```python
from build123d import *

# Parameters (mm, degrees)
SKETCH1_R                                         = 57.5
BOSS_EXTRUDE1_DEPTH                               = 6.4
SKETCH2_W                                         = 25.525
SKETCH2_H                                         = 20.295
CUT_EXTRUDE1_DEPTH                                = 7.4
SKETCH3_W                                         = 4
SKETCH3_H                                         = 20.295
CUT_EXTRUDE2_DEPTH                                = 3
CUT_EXTRUDE3_DEPTH                                = 3
SKETCH5_R                                         = 1
CUT_EXTRUDE4_DEPTH                                = 7.4
CSK_FOR_8_FLAT_HEAD_SOCKET_CAP_SCREW1_D           = 4.9149
CSK_FOR_8_FLAT_HEAD_SOCKET_CAP_SCREW1_CSINK_D     = 9.1186
CSK_FOR_8_FLAT_HEAD_SOCKET_CAP_SCREW1_CSINK_ANGLE = 82
BOSS_EXTRUDE2_DEPTH                               = 6.4
FILLET1_R                                         = 2
SKETCH10_R                                        = 57.5
SKETCH10_R_2                                      = 54.5
BOSS_EXTRUDE3_DEPTH                               = 6.375
FILLET2_R                                         = 1


with BuildPart() as part:
    # Sketch1 → Boss-Extrude1 (new body)
    with BuildSketch(Plane(origin=(0, 0, 0), x_dir=(1, 0, 0), z_dir=(0, 1, 0))):
        Circle(SKETCH1_R)
        with BuildLine():
            Line((-17.49944642, 27), (17.49944642, 27))
            ThreePointArc((17.49944642, 27), (32.175, 0), (17.49944642, -27))
            Line((17.49944642, -27), (-17.49944642, -27))
            ThreePointArc((-17.49944642, -27), (-32.175, 0), (-17.49944642, 27))
        make_face(mode=Mode.SUBTRACT)
    extrude(amount=BOSS_EXTRUDE1_DEPTH)

    # Sketch2 → Cut-Extrude1 (cut, through all)
    with BuildSketch(Plane(origin=(0, 6.4, 0), x_dir=(1, 0, 0), z_dir=(0, 1, 0))):
        with Locations((0, 40.1475)):
            Rectangle(SKETCH2_W, SKETCH2_H)
        with Locations((0, -40.1475)):
            Rectangle(SKETCH2_W, SKETCH2_H)
    extrude(amount=-CUT_EXTRUDE1_DEPTH, mode=Mode.SUBTRACT)

    # Sketch3 → Cut-Extrude2 (cut)
    with BuildSketch(Plane.XZ):
        with Locations((14.7625, 40.1475)):
            Rectangle(SKETCH3_W, SKETCH3_H)
        with Locations((-14.7625, 40.1475)):
            Rectangle(SKETCH3_W, SKETCH3_H)
        with Locations((14.7625, -40.1475)):
            Rectangle(SKETCH3_W, SKETCH3_H)
        with Locations((-14.7625, -40.1475)):
            Rectangle(SKETCH3_W, SKETCH3_H)
    extrude(amount=-CUT_EXTRUDE2_DEPTH, mode=Mode.SUBTRACT)

    # Sketch4 → Cut-Extrude3 (cut)
    with BuildSketch(Plane.XZ):
        with BuildLine():
            Line((-19.770159359, 30.503496503), (-17.49944642, 27))
            ThreePointArc((-17.49944642, 27), (-32.175, 0), (-17.49944642, -27))
            Line((-17.49944642, -27), (-19.770159359, -30.503496503))
            ThreePointArc((-19.770159359, -30.503496503), (-36.35, 0), (-19.770159359, 30.503496503))
        make_face()
        with BuildLine():
            ThreePointArc((19.770159359, 30.503496503), (36.35, 0), (19.770159359, -30.503496503))
            Line((19.770159359, -30.503496503), (17.49944642, -27))
            ThreePointArc((17.49944642, -27), (32.175, 0), (17.49944642, 27))
            Line((17.49944642, 27), (19.770159359, 30.503496503))
        make_face()
    extrude(amount=-CUT_EXTRUDE3_DEPTH, mode=Mode.SUBTRACT)

    # Sketch5 → Cut-Extrude4 (cut, through all)
    with BuildSketch(Plane.XZ):
        with Locations((-33.941125497, 33.941125497)):
            Circle(SKETCH5_R)
        with Locations((33.941125497, 33.941125497)):
            Circle(SKETCH5_R)
        with Locations((33.941125497, -33.941125497)):
            Circle(SKETCH5_R)
        with Locations((-33.941125497, -33.941125497)):
            Circle(SKETCH5_R)
    extrude(amount=-CUT_EXTRUDE4_DEPTH, mode=Mode.SUBTRACT)

    # CSK for #8 Flat Head Socket Cap Screw1 (through all)
    with Locations(Plane(origin=(0, 6.4, 0), x_dir=(1, 0, 0), z_dir=(0, 1, 0))):
        with Locations((-33.941125497, 33.941125497), (33.941125497, 33.941125497), (33.941125497, -33.941125497), (-33.941125497, -33.941125497)):
            CounterSinkHole(CSK_FOR_8_FLAT_HEAD_SOCKET_CAP_SCREW1_D / 2, CSK_FOR_8_FLAT_HEAD_SOCKET_CAP_SCREW1_CSINK_D / 2, counter_sink_angle=CSK_FOR_8_FLAT_HEAD_SOCKET_CAP_SCREW1_CSINK_ANGLE)

    # Sketch9 → Boss-Extrude2 (add)
    with BuildSketch(Plane(origin=(0, 6.4, 0), x_dir=(1, 0, 0), z_dir=(0, 1, 0))):
        with BuildLine():
            Line((-17.49944642, 27), (17.49944642, 27))
            Line((17.49944642, 27), (9.178880504, 22.337651011))
            ThreePointArc((9.178880504, 22.337651011), (0, 24.15), (-9.178880504, 22.337651011))
            Line((-9.178880504, 22.337651011), (-17.49944642, 27))
        make_face()
        with BuildLine():
            Line((17.49944642, -27), (9.178880504, -22.337651011))
            ThreePointArc((9.178880504, -22.337651011), (0, -24.15), (-9.178880504, -22.337651011))
            Line((-9.178880504, -22.337651011), (-17.49944642, -27))
            Line((-17.49944642, -27), (17.49944642, -27))
        make_face()
    extrude(amount=-BOSS_EXTRUDE2_DEPTH)

    # Fillet1
    fillet1_edges = [part.edges().sort_by_distance(p)[0] for p in [
        (9.178880504, 3.2, -22.337651011),
        (-9.178880504, 3.2, -22.337651011),
        (-9.178880504, 3.2, 22.337651011),
        (9.178880504, 3.2, 22.337651011),
        (-57.5, 6.4, 0),
    ]]
    fillet(fillet1_edges, radius=FILLET1_R)

    # Sketch10 → Boss-Extrude3 (add)
    with BuildSketch(Plane.XZ):
        Circle(SKETCH10_R)
        Circle(SKETCH10_R_2, mode=Mode.SUBTRACT)
    extrude(amount=BOSS_EXTRUDE3_DEPTH)

    # Fillet2
    fillet2_edges = [part.edges().sort_by_distance(p)[0] for p in [
        (-54.5, -6.375, 0),
    ]]
    fillet(fillet2_edges, radius=FILLET2_R)


solid = part.part
```
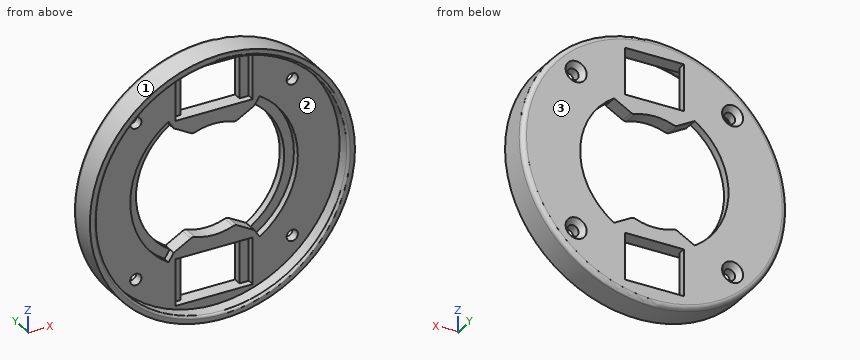
The model under review builds one solid part; all positions refer to its coordinate system, in mm. Face numbers are marked on the shaded views. Round coordinates to 2 decimals unless told otherwise and drop trailing zeros. Write each loop counter-clockwise with the first axis right and the second up, starting at its lowest first coordinate (ties: lowest second). Pieces come first, ordered by that corner, then holes.
(1) Wall thickness on L1, parallel to Z at x = 0, y = -4.2; L2, parallel to Z at x = 15, y = 0.5 (3 decimals); L3, parallel to Z at x = -33, y = 2: over which ranges is each line inside the solid? List them lowest first.
(2) We need section A-A on z = 0. Give the boundary of the cut face in (x, y) (3 decimals), and give its area (3 significant figures).
(3) Insertion check: pin 1 (2.5 mm diameter, centred on y = 1, z = 44.5, fed in from -X); pin 2 (8 mm diameter, centred on x = 33.94, z = -33.94, fed in from -Y); pin 3 (1.9 mm diameter, centred on x = -5, y = 4, fed in from +Z). Each pin has a flat end and moves straight along its axis. Give the tip position at first contact, or say it passes through.
(4) We need section B-B on x = 0. Give the boundary of the cut face in (y, z) (3 decimals), and give its area (3 significant figures).
(5) We need section C-C on x = -35. Give the number of separate pieces and of enclosed holes in the cut face, and give its area (3 significant figures).
(6) Mouldability with a two-part tool opening along Z and no side actions: class the marked faces 1, 2 and 3 as +Z half, -Z half, draft (parallel to the pull), parting line (faces both ways), or undercut.
Findings below:
1. L1: z = -57.5 to -54.5, 54.5 to 57.5
1. L2: z = -55.509 to -50.295, -30 to -25.599, 25.599 to 30, 50.295 to 55.509
1. L3: z = -47.09 to -36.21, -31.67 to -15.24, 15.24 to 31.67, 36.21 to 47.09
2. outline: (-57.5, -6.375) - (-55.5, -6.375) arc R1 ccw to (-54.5, -5.375) - (-54.5, 0) - (-36.35, 0) - (-36.35, 3) - (-32.175, 3) - (-32.175, 6.4) - (-55.5, 6.4) arc R2 ccw to (-57.5, 4.4) - close; (32.175, 3) - (36.35, 3) - (36.35, 0) - (54.5, 0) - (54.5, -5.375) arc R1 ccw to (55.5, -6.375) - (57.5, -6.375) - (57.5, 4.4) arc R2 ccw to (55.5, 6.4) - (32.175, 6.4) - close
2. area: 335 mm2
3. pin 1: stops at x = -37.89
3. pin 2: stops at y = 0
3. pin 3: stops at z = 57.36
4. outline: (-6.375, -57.5) - (4.4, -57.5) arc R2 ccw to (6.4, -55.5) - (6.4, -50.295) - (0, -50.295) - (0, -54.5) - (-5.375, -54.5) arc R1 ccw to (-6.375, -55.5) - close; (-6.375, 55.5) arc R1 ccw to (-5.375, 54.5) - (0, 54.5) - (0, 50.295) - (6.4, 50.295) - (6.4, 55.5) arc R2 ccw to (4.4, 57.5) - (-6.375, 57.5) - close; (0, -30) - (6.4, -30) - (6.4, -24.15) - (0, -24.15) - close; (0, 24.15) - (6.4, 24.15) - (6.4, 30) - (0, 30) - close
4. area: 203 mm2
5. separate pieces: 3
5. enclosed holes: 0
5. area: 504 mm2
6. face 1: parting line
6. face 2: undercut
6. face 3: draft
